Autodesk Inventor part; units mm, degrees
ref_plane "YZ Plane" through (0, 0, 0) normal (1, 0, 0) x (0, 1, 0)
ref_plane "XZ Plane" through (0, 0, 0) normal (0, 1, 0) x (-1, 0, 0)
ref_plane "XY Plane" through (0, 0, 0) normal (0, 0, 1) x (1, 0, 0)
sketch "Sketch2" plane through (0, 0, 0) normal (0, 0, 1) x (1, 0, 0)
  line L0 (0, 0) -> (0, 8.357) construction
  line L1 (0, 0) -> (2.8603, 0) construction
  arc A0 (-0.3969, 4.8591) -> (-0.71, 3.0831) centre (1.785, 3.5588) ccw
  arc A1 (0.71, 3.0831) -> (0.3969, 4.8591) centre (-1.785, 3.5588) ccw
  line L2 (0.3969, 4.8591) -> (-0.3969, 4.8591)
  line L3 (-0.71, 3.0831) -> (0.71, 3.0831) construction
  arc A2 (0.71, 3.0831) -> (0.3969, 4.8591) centre (-1.785, 3.5588) ccw
  line L4 (0.3969, 4.8591) -> (-0.3969, 4.8591)
  arc A3 (-0.3969, 4.8591) -> (-0.71, 3.0831) centre (1.785, 3.5588) ccw
  line L5 (0.3969, 4.8591) -> (0.71, 3.0831) construction
  arc A4 (-1.678, 2.6822) -> (-3.1553, 3.7166) centre (-3.7786, 1.2542) ccw
  line L6 (-3.1553, 3.7166) -> (-3.7166, 3.1553)
  arc A5 (-3.7166, 3.1553) -> (-2.6822, 1.678) centre (-1.2542, 3.7786) ccw
  arc A6 (-3.0831, 0.71) -> (-4.8591, 0.3969) centre (-3.5588, -1.785) ccw
  line L7 (-4.8591, 0.3969) -> (-4.8591, -0.3969)
  arc A7 (-4.8591, -0.3969) -> (-3.0831, -0.71) centre (-3.5588, 1.785) ccw
  arc A8 (-2.6822, -1.678) -> (-3.7166, -3.1553) centre (-1.2542, -3.7786) ccw
  line L8 (-3.7166, -3.1553) -> (-3.1553, -3.7166)
  arc A9 (-3.1553, -3.7166) -> (-1.678, -2.6822) centre (-3.7786, -1.2542) ccw
  arc A10 (-0.71, -3.0831) -> (-0.3969, -4.8591) centre (1.785, -3.5588) ccw
  line L9 (-0.3969, -4.8591) -> (0.3969, -4.8591)
  arc A11 (0.3969, -4.8591) -> (0.71, -3.0831) centre (-1.785, -3.5588) ccw
  arc A12 (1.678, -2.6822) -> (3.1553, -3.7166) centre (3.7786, -1.2542) ccw
  line L10 (3.1553, -3.7166) -> (3.7166, -3.1553)
  arc A13 (3.7166, -3.1553) -> (2.6822, -1.678) centre (1.2542, -3.7786) ccw
  arc A14 (3.0831, -0.71) -> (4.8591, -0.3969) centre (3.5588, 1.785) ccw
  line L11 (4.8591, -0.3969) -> (4.8591, 0.3969)
  arc A15 (4.8591, 0.3969) -> (3.0831, 0.71) centre (3.5588, -1.785) ccw
  arc A16 (2.6822, 1.678) -> (3.7166, 3.1553) centre (1.2542, 3.7786) ccw
  line L12 (3.7166, 3.1553) -> (3.1553, 3.7166)
  arc A17 (3.1553, 3.7166) -> (1.678, 2.6822) centre (3.7786, 1.2542) ccw
  line L13 (-1.678, 2.6822) -> (-0.71, 3.0831) construction
  arc A18 (-0.71, 3.0831) -> (-1.678, 2.6822) centre (0, 0) ccw
  arc A19 (1.678, 2.6822) -> (0.71, 3.0831) centre (0, 0) ccw
  arc A20 (3.0831, 0.71) -> (2.6822, 1.678) centre (0, 0) ccw
  arc A21 (2.6822, -1.678) -> (3.0831, -0.71) centre (0, 0) ccw
  arc A22 (0.71, -3.0831) -> (1.678, -2.6822) centre (0, 0) ccw
  arc A23 (-1.678, -2.6822) -> (-0.71, -3.0831) centre (0, 0) ccw
  arc A24 (-2.6822, 1.678) -> (-3.0831, 0.71) centre (0, 0) ccw
  arc A25 (-3.0831, -0.71) -> (-2.6822, -1.678) centre (0, 0) ccw
  point P0 (0, 4.8591)
  point P1 (-3.4359, 3.4359)
  point P2 (-4.8591, 0)
  point P3 (-3.4359, -3.4359)
  point P4 (0, -4.8591)
  point P5 (3.4359, -3.4359)
  point P6 (4.8591, 0)
  point P7 (3.4359, 3.4359)
  dimension "d11" = 0.7937
  dimension "d13" = 2.54
  dimension "d14" = 80
  dimension "d15" = 1.8034
  dimension "d18" = 360
  dimension "d20" = 1.0477
extrude "Extrusion2" add sketch "Sketch2" along normal blind 1.5875
properties part number "Planet"
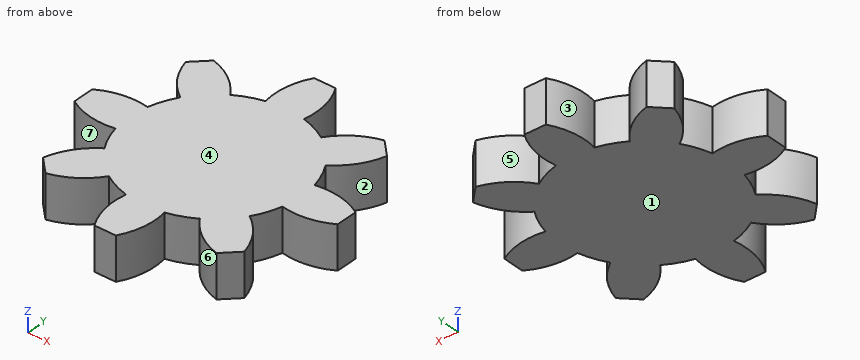
Design review of the part built by this model. Coordinates are the model's own, in mm. Face numbers are marked on the shaded views. A direction names the side the tool comes from. Give positions to 0.01 mm unless a question says otherwise; leave off trailing zeros. Loops run counter-clockwise (first coordinate to the right, second up) from the corner with the lowest first, then second, coordinate; pieces in that order, holes last. Notation, with made-up numbers: (-23.5, 80) -> (24.5, 80) arc R29 cw to (24.5, 115) -> close; hole circle Ø6 at (20, 55.25). An arc over 180 degrees is marked (long way). One line per question, with ' | ' between items. Start each with the question number.
(1) We need section B-B (x = -1.25). State the section outline as (y, z) points, and give its area (3 significant figures).
(2) Draft analysis for pull direction X (two halves, no side actions). For the marked faces 1, 2 and 3, state which applies: +X half, -X half, draft (parallel to the pull), parting line (faces both ways), or undercut.
(3) For the marked faces 4, 5, 6 and 7, list the 3-axis set-ups (+Z, -Z, +X, -X, +Y, -Y) from which the entire face can be reached by the end or side of a thin tool; tool diameter is ignored.
(4) For line 1 (Y direction, x = -3.5, z = 1.2); line 2 (X direction, y = 0.5, z = 0.2); line 3 (X direction, y = -4.5, z = 0.3), list the stretches that pass through material, from the lowest coordinate up.
(5) Insertion check: P1, Ø5, axis at x = 2, y = 2, coming from the -Z side. The pin has a flat end and moves straight along its axis. Give the tip position at first contact, or say it passes through.
(6) We need section C-C (y = -1.5). State the section outline as (x, z) points.
The answers:
1) outline: (-2.91, 0) -> (2.91, 0) -> (2.91, 1.59) -> (-2.91, 1.59) -> close | area: 9.23 mm^2
2) face 1: draft | face 2: +X half | face 3: undercut
3) face 4: +Z, +X, -X, +Y, -Y | face 5: +Z, -Z, +Y | face 6: +Z, -Z, -Y | face 7: +Z, -Z
4) line 1: y = -3.37 to -2.59, -0.75 to 0.75, 2.59 to 3.37 | line 2: x = -4.67 to 4.67 | line 3: x = -0.57 to 0.57
5) P1: stops at z = 0
6) outline: (-2.79, 0) -> (2.79, 0) -> (2.79, 1.59) -> (-2.79, 1.59) -> close
